```python
from build123d import *

# Parameters (mm, degrees)
SKETCH2_R                = 1.5
BOSS_EXTRUDE1_DEPTH      = 600
BOSS_EXTRUDE2_DEPTH      = 1.5
BOSS_EXTRUDE2_DEPTH_BACK = 1.5
SKETCH3_R                = 7.5
BOSS_EXTRUDE3_DEPTH      = 1.5


with BuildPart() as part:
    # Sketch2 → Boss-Extrude1 (new body)
    with BuildSketch(Plane(origin=(0, 0, -600), x_dir=(-1, 0, 0), z_dir=(0, 0, -1))):
        Circle(SKETCH2_R)
    extrude(amount=-BOSS_EXTRUDE1_DEPTH)

    # Sketch1 → Boss-Extrude2 (add, two sides: drawn at the far end of the back side and taken through both)
    with BuildSketch(Plane(origin=(0, 0, 0), x_dir=(0, 0, -1), z_dir=(1, 0, 0)).offset(-BOSS_EXTRUDE2_DEPTH_BACK)):
        Polygon((0, 0), (0, -1.5), (-3, -1.5), (-3, 353), (603, 353), (603, -1.5), (600, -1.5), (600, 0), (600, 350), (0, 350), align=None)
    extrude(amount=BOSS_EXTRUDE2_DEPTH + BOSS_EXTRUDE2_DEPTH_BACK)

    # Sketch3 → Boss-Extrude3 (add)
    with BuildSketch(Plane(origin=(0, 0, -25), x_dir=(-1, 0, 0), z_dir=(0, 0, -1))):
        Polygon((-1.5, 350), (-1.5, 353), (-51.5, 353), (-51.5, 375), (-76.5, 375), (-76.5, 350), align=None)
        with Locations(Location((-64, 362.5, 0), (0, 0, 90))):
            Circle(SKETCH3_R, mode=Mode.SUBTRACT)
    extrude(amount=BOSS_EXTRUDE3_DEPTH)


solid = part.part
```
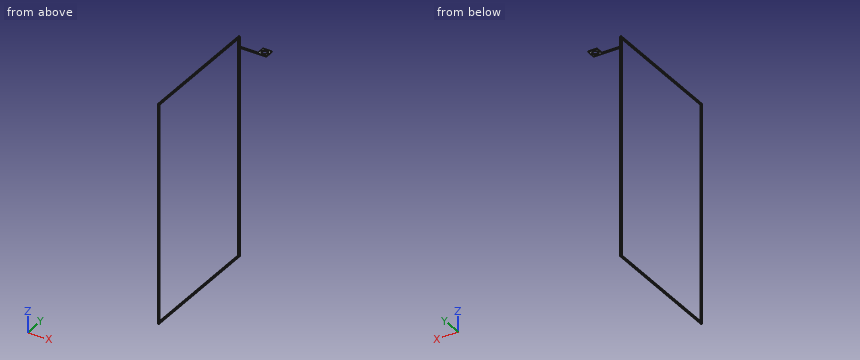
Geometry check sheet. Reference: the model listing, model coordinates, mm. Coordinates: 2 decimals unless noted, no trailing zeros. Order: outer loops, then holes, each group sorted by start corner. A loop starts at its lowest first (then second) coordinate and runs counter-clockwise, first axis right, second up. Notation, with made-up numbers: M -32,53.25 L 22,53.25 A11 cw 22,62.25 Z; hole C 49.5,18 d6. An arc over 180 degrees is marked long. One line per question, with ' | ' between items. Start each with the question number.
Item 1: Cross-section at C-C on z = -80.5. Enter the section's corners in (x, y), then the cut area to 3 significant figures.
Item 2: Cross-section at B-B on y = 362.5. Enter the section's corners in (x, z).
Item 3: Gauge pin test, flat ends, axial feed: pin 1 (7.5 mm diameter, centred on x = 56, y = 362.5, fed in from +Z); pin 2 (19.5 mm diameter, centred on x = 64, y = 362.5, fed in from -Z); pin 3 (1.6 mm diameter, centred on y = 367, z = -25.5, fed in from -X). Record the tip position at first contact, or that the pin passes through.
Item 4: Material ranges on L1, parallel to X at y = 362.5, z = -25.35, recorded low to high. Write a range as [from, to].
Item 5: Cross-section at D-D on x = 31.5. Enter the section's corners in (y, z).
Item 6: Cross-section at A-A on x = 64. Enter the section's corners in (y, z).
Findings:
1) outline: C 0,0 d3; M -1.5,350 L 1.5,350 L 1.5,353 L -1.5,353 Z | area: 16.1 mm²
2) outline: M 51.5,-26.5 L 56.5,-26.5 L 56.5,-25 L 51.5,-25 Z; M 71.5,-26.5 L 76.5,-26.5 L 76.5,-25 L 71.5,-25 Z
3) pin 1: stops at z = -25 | pin 2: stops at z = -26.5 | pin 3: stops at x = 51.5
4) L1: x = [51.5, 56.5], [71.5, 76.5]
5) outline: M 350,-26.5 L 353,-26.5 L 353,-25 L 350,-25 Z
6) outline: M 350,-26.5 L 355,-26.5 L 355,-25 L 350,-25 Z; M 370,-26.5 L 375,-26.5 L 375,-25 L 370,-25 Z
